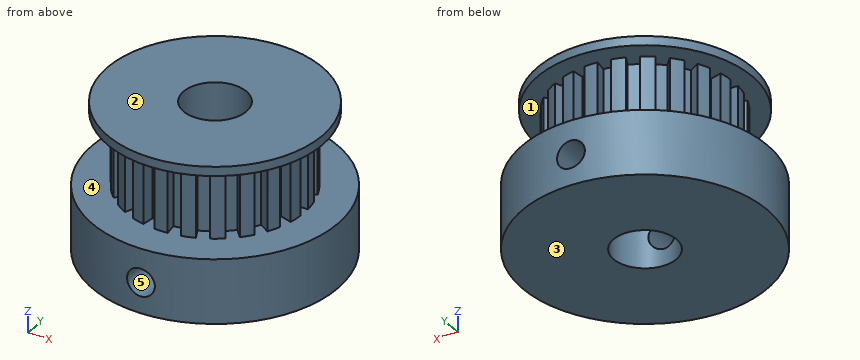
```python
from build123d import *

# Parameters (mm, degrees)
SKETCH1_R               = 8.89
BOSS_EXTRUDE1_DEPTH     = 0.762
SKETCH2_R               = 7.366
BOSS_EXTRUDE2_DEPTH     = 6.096
SKETCH3_R               = 10.16
BOSS_EXTRUDE3_DEPTH     = 5.334
SKETCH4_R               = 2.6035
CUT_EXTRUDE1_DEPTH      = 25.654
SKETCH5_W               = 6.096
SKETCH5_H               = 1.016
CUT_EXTRUDE2_DEPTH      = 1.016
CIRPATTERN1_COUNT       = 22
SKETCH6_R               = 1.143
CUT_EXTRUDE3_DEPTH      = 22.098
CUT_EXTRUDE3_DEPTH_BACK = 22.098


with BuildPart() as part:
    # Sketch1 → Boss-Extrude1 (new body)
    with BuildSketch(Plane.XY):
        Circle(SKETCH1_R)
    extrude(amount=-BOSS_EXTRUDE1_DEPTH)

    # Sketch2 → Boss-Extrude2 (add)
    with BuildSketch(Plane(origin=(0, 0, -0.762), x_dir=(-1, 0, 0), z_dir=(0, 0, -1))):
        Circle(SKETCH2_R)
    extrude(amount=BOSS_EXTRUDE2_DEPTH)

    # Sketch3 → Boss-Extrude3 (add)
    with BuildSketch(Plane(origin=(0, 0, -6.858), x_dir=(-1, 0, 0), z_dir=(0, 0, -1))):
        Circle(SKETCH3_R)
    extrude(amount=BOSS_EXTRUDE3_DEPTH)

    # Sketch4 → Cut-Extrude1 (cut)
    with BuildSketch(Plane.XY):
        Circle(SKETCH4_R)
    extrude(amount=-CUT_EXTRUDE1_DEPTH, mode=Mode.SUBTRACT)

    # Sketch5 → Cut-Extrude2 (cut)
    with BuildSketch(Plane.ZY.offset(7.366)):
        with Locations((-3.81, 0)):
            Rectangle(SKETCH5_W, SKETCH5_H)
    cut_extrude2 = extrude(amount=-CUT_EXTRUDE2_DEPTH, mode=Mode.SUBTRACT)

    # CirPattern1: Cut-Extrude2 ×22 about axis
    cirpattern1_axis = Axis((0, 0, 0), (0, 0, 1))
    for i in range(1, CIRPATTERN1_COUNT):
        add(cut_extrude2.rotate(cirpattern1_axis, i * 360 / CIRPATTERN1_COUNT), mode=Mode.SUBTRACT)

    # Sketch6 → Cut-Extrude3 (cut, two sides)
    with BuildSketch(Plane(origin=(0, 0, 0), x_dir=(1, 0, 0), z_dir=(0, 1, 0))) as cut_extrude3_sk:
        with Locations((0, 9.652)):
            Circle(SKETCH6_R)
    extrude(amount=CUT_EXTRUDE3_DEPTH, mode=Mode.SUBTRACT)
    extrude(cut_extrude3_sk.sketch, amount=-CUT_EXTRUDE3_DEPTH_BACK, mode=Mode.SUBTRACT)


solid = part.part
```
The listing builds one solid part. Answer for the finished solid, in the listing's coordinates (mm). Face numbers are marked on the shaded views. A direction names the side the tool comes from. Give positions to 0.01 mm unless a question says otherwise; leave off trailing zeros. Write each loop counter-clockwise with the first axis right and the second up, starting at its lowest first coordinate (ties: lowest second). Pieces come first, ordered by that corner, then holes. Notation, with made-up numbers: (12, 3.25) -> (23, 3.25) arc R11 ccw to (23, 17.25) -> close; hole circle Ø10 at (84, -26.5). An arc over 180 degrees is marked (long way). Write item = value, one per line. Start each with the question number.
1) The part is cut by section A-A, the plane y = 0. Determine the outline of the cut face in (x, z).
2) Determine the mould class of the marked faces 1, 2 and 3 for opening direction Z: +Z half, -Z half, draft (parallel to the pull), parting line (faces both ways), or undercut.
3) Which of the six approach directions +Z, -Z, +X, -X, +Y, -Y give full straight-line access (tool end or side, diameter ignored) to the marked faces 4 and 5?
4) The part is cut by section D-D, the plane z = -10. Determine the outline of the cut face in (x, y).
5) Straight lines are drawn through the part: line 1 along Z through (x, y) = (0, 8.75) (3 decimals); line 2 along Y through (x, z) = (-0.25, -6); line 3 along Z through (x, y) = (-2, 8.5). For each, find the intervals that lie inside material, in ascending order.
6) The part is cut by section C-C, the plane y = 7.75. Determine the outline of the cut face in (x, z), and give its area (3 significant figures).
7) The part is cut by section B-B, the plane x = 0. Determine the outline of the cut face in (y, z) (1 decimal), and give its area (3 significant figures).
8) Each of these flat-tipped pins is pushed along its axis until it touches: pin 1 (1.1 mm diameter, centred on y = 0, z = -2.5, fed in from -X); pin 2 (10 mm diameter, centred on x = 5.5, y = 4, fed in from +Z); pin 3 (1.5 mm diameter, centred on y = -4.5, z = -6.5, fed in from +X); pin 4 (3 mm diameter, centred on x = 0, y = 0, fed in from -Z). Where does it stop, or does it pass through?
Solutions:
q1.outline = (-10.16, -12.19) -> (-2.6, -12.19) -> (-2.6, 0) -> (-8.89, 0) -> (-8.89, -0.76) -> (-6.35, -0.76) -> (-6.35, -6.86) -> (-10.16, -6.86) -> close; (2.6, -12.19) -> (10.16, -12.19) -> (10.16, -6.86) -> (6.35, -6.86) -> (6.35, -0.76) -> (8.89, -0.76) -> (8.89, 0) -> (2.6, 0) -> close
q2.face_1 = undercut
q2.face_2 = +Z half
q2.face_3 = -Z half
q3.face_4 = none
q3.face_5 = +Y, -Y
q4.outline = (-1.09, -10.1) -> (-1.09, -2.36) arc R2.6 cw to (-1.09, 2.36) -> (-1.09, 10.1) arc R10.16 ccw to start; (1.09, -10.1) arc R10.16 ccw to (1.09, 10.1) -> (1.09, 2.36) arc R2.6 cw to (1.09, -2.36) -> close
q5.line_1 = -12.192 to -10.795, -8.509 to -6.858, -0.762 to 0
q5.line_2 = -7.36 to -2.59, 2.59 to 7.36
q5.line_3 = -12.19 to -6.86, -0.76 to 0
q6.outline = (-6.57, -12.19) -> (6.57, -12.19) -> (6.57, -6.86) -> (-6.57, -6.86) -> close; (-4.36, -0.76) -> (4.36, -0.76) -> (4.36, 0) -> (-4.36, 0) -> close; hole circle Ø2.29 at (0, -9.65)
q6.area = 72.6 mm²
q7.outline = (-10.2, -12.2) -> (-2.6, -12.2) -> (-2.6, -10.8) -> (-10.2, -10.8) -> close; (-10.2, -8.5) -> (-2.6, -8.5) -> (-2.6, 0) -> (-8.9, 0) -> (-8.9, -0.8) -> (-7.4, -0.8) -> (-7.4, -6.9) -> (-10.2, -6.9) -> close; (2.6, -12.2) -> (10.2, -12.2) -> (10.2, -10.8) -> (2.6, -10.8) -> close; (2.6, -8.5) -> (10.2, -8.5) -> (10.2, -6.9) -> (7.4, -6.9) -> (7.4, -0.8) -> (8.9, -0.8) -> (8.9, 0) -> (2.6, 0) -> close
q7.area = 114 mm²
q8.pin_1 = -7.35
q8.pin_2 = 0
q8.pin_3 = 9.41
q8.pin_4 = through
